Verification items for the finished model (mm, model axes). A direction names the side the tool comes from. Give positions to 0.01 mm unless a question says otherwise; leave off trailing zeros. Loops run counter-clockwise (first coordinate to the right, second up) from the corner with the lowest first, then second, coordinate; pieces in that order, holes last. Notation, with made-up numbers: (46.25, 35.5) - (74.25, 35.5) arc R36 ccw to (74.25, 71.5) - close; hole circle Ø7 at (59, 70.25). An arc over 180 degrees is marked (long way). One line per question, with ' | ' between items. Start each with the question number.
1. Mould release check, pull along X, two halves, no side actions. Record for faces 5 (the face through (10, 175.4, 9.7)), 6 (the face through (-7, 178, -9.5)), 7 (the face through (0, 169, -10)): +X half, -X half, draft (parallel to the pull), parting line (faces both ways), or undercut.
2. Section check B-B, the plane z = 0. Enter the section's corners in (x, y).
3. Section check C-C, the plane y = 100.5. Enter the section's corners in (x, z), then the cut area to 3 significant figures.
4. Section check A-A, the plane y = 174. Enter the section's corners in (x, z).
5. Tool access check on faces 1 (the face through (-7.81, 75.92, -1.73)), 2 (the face through (7, 178, -9.5)), 3 (the face through (-2.4, 173.8, 9)), 4 (the face through (-7.81, 173.76, -1.73)). Record the directions out of +Z, -Z, +X, -X, +Y, -Y that give a thin tool (end or side, any length) a straight path to the whole face; none if there is none.
6. Thickness scan on line 1 along Y through (x, z) = (0, -9.5); line 2 along X through (y, z) = (73, 0); line 3 along X through (y, z) = (155, -1). Record the ranges inside material, lowest first. Write a range as from..to.
7. Depth check by flat-ended pin: pin 1 Ø6 at (x, y) = (2.5, 109) entering from +Z; pin 2 Ø3 at (x, y) = (0, 31.5) entering from -Z; pin 3 Ø9 at (x, z) = (4, 2) entering from +Y; pin 4 Ø4 at (y, z) = (118, -3) entering from -X. Enter the tip coordinate at first touch or a pass-through.
from build123d import *

# Parameters (mm, degrees)
SKETCH1_R           = 8
BOSS_EXTRUDE1_DEPTH = 154
SKETCH2_W           = 20
SKETCH2_H           = 20
BOSS_EXTRUDE2_DEPTH = 40
SKETCH3_W           = 18
SKETCH3_H           = 34
CUT_EXTRUDE1_DEPTH  = 196.28440798
SKETCH6_R           = 8
BOSS_EXTRUDE3_DEPTH = 34
SKETCH7_R           = 3.5
CUT_EXTRUDE4_DEPTH  = 1
CUT_EXTRUDE5_DEPTH  = 1
SKETCH4_R           = 6
CUT_EXTRUDE3_DEPTH  = 195.514780929


with BuildPart() as part:
    # Sketch1 → Boss-Extrude1 (new body)
    with BuildSketch(Plane(origin=(0, 0, 0), x_dir=(1, 0, 0), z_dir=(0, 1, 0))):
        with Locations(Location((0, 0, 0), (0, 0, 270))):
            Circle(SKETCH1_R)
    extrude(amount=BOSS_EXTRUDE1_DEPTH)

    # Sketch2 → Boss-Extrude2 (add)
    with BuildSketch(Plane(origin=(0, 154, 0), x_dir=(1, 0, 0), z_dir=(0, 1, 0))):
        Rectangle(SKETCH2_W, SKETCH2_H)
    extrude(amount=BOSS_EXTRUDE2_DEPTH)

    # Sketch3 → Cut-Extrude1 (cut, through all)
    with BuildSketch(Plane.ZY.offset(10)):
        with Locations((0, 174)):
            Rectangle(SKETCH3_W, SKETCH3_H)
    extrude(amount=-CUT_EXTRUDE1_DEPTH, mode=Mode.SUBTRACT)

    # Sketch6 → Boss-Extrude3 (add)
    with BuildSketch(Plane(origin=(0, 157, 0), x_dir=(1, 0, 0), z_dir=(0, 1, 0))):
        with Locations(Location((0, 0, 0), (0, 0, 270))):
            Circle(SKETCH6_R)
    extrude(amount=BOSS_EXTRUDE3_DEPTH)

    # Sketch7 → Cut-Extrude4 (cut)
    with BuildSketch(Plane(origin=(0, 0, -10), x_dir=(-1, 0, 0), z_dir=(0, 0, -1))):
        with Locations((0, 174)):
            Circle(SKETCH7_R)
        with BuildLine():
            Line((-0.25, 178), (0.25, 178))
            ThreePointArc((0.25, 178), (0.780330086, 178.219669914), (1, 178.75))
            Line((1, 178.75), (1, 185.25))
            ThreePointArc((1, 185.25), (0.780330086, 185.780330086), (0.25, 186))
            Line((0.25, 186), (-0.25, 186))
            ThreePointArc((-0.25, 186), (-0.780330086, 185.780330086), (-1, 185.25))
            Line((-1, 185.25), (-1, 178.75))
            ThreePointArc((-1, 178.75), (-0.780330086, 178.219669914), (-0.25, 178))
        make_face()
        with BuildLine():
            Line((-4.4, 176.05), (-9.6, 179.95))
            ThreePointArc((-9.6, 179.95), (-9.89246212, 180.443933983), (-9.75, 181))
            Line((-9.75, 181), (-9.45, 181.4))
            ThreePointArc((-9.45, 181.4), (-8.956066017, 181.69246212), (-8.4, 181.55))
            Line((-8.4, 181.55), (-3.2, 177.65))
            ThreePointArc((-3.2, 177.65), (-2.90753788, 177.156066017), (-3.05, 176.6))
            Line((-3.05, 176.6), (-3.35, 176.2))
            ThreePointArc((-3.35, 176.2), (-3.843933983, 175.90753788), (-4.4, 176.05))
        make_face()
        with BuildLine():
            Line((3.2, 177.65), (8.4, 181.55))
            ThreePointArc((8.4, 181.55), (8.956066017, 181.69246212), (9.45, 181.4))
            Line((9.45, 181.4), (9.75, 181))
            ThreePointArc((9.75, 181), (9.89246212, 180.443933983), (9.6, 179.95))
            Line((9.6, 179.95), (4.4, 176.05))
            ThreePointArc((4.4, 176.05), (3.843933983, 175.90753788), (3.35, 176.2))
            Line((3.35, 176.2), (3.05, 176.6))
            ThreePointArc((3.05, 176.6), (2.90753788, 177.156066017), (3.2, 177.65))
        make_face()
        with BuildLine():
            Line((3.35, 263.8), (3.05, 263.4))
            ThreePointArc((3.05, 263.4), (2.90753788, 262.843933983), (3.2, 262.35))
            Line((3.2, 262.35), (8.4, 258.45))
            ThreePointArc((8.4, 258.45), (8.956066017, 258.30753788), (9.45, 258.6))
            Line((9.45, 258.6), (9.75, 259))
            ThreePointArc((9.75, 259), (9.89246212, 259.556066017), (9.6, 260.05))
            Line((9.6, 260.05), (4.4, 263.95))
            ThreePointArc((4.4, 263.95), (3.843933983, 264.09246212), (3.35, 263.8))
        make_face()
        with BuildLine():
            Line((-3.05, 263.4), (-3.35, 263.8))
            ThreePointArc((-3.35, 263.8), (-3.843933983, 264.09246212), (-4.4, 263.95))
            Line((-4.4, 263.95), (-9.6, 260.05))
            ThreePointArc((-9.6, 260.05), (-9.89246212, 259.556066017), (-9.75, 259))
            Line((-9.75, 259), (-9.45, 258.6))
            ThreePointArc((-9.45, 258.6), (-8.956066017, 258.30753788), (-8.4, 258.45))
            Line((-8.4, 258.45), (-3.2, 262.35))
            ThreePointArc((-3.2, 262.35), (-2.90753788, 262.843933983), (-3.05, 263.4))
        make_face()
        with BuildLine():
            Line((1, 261.25), (1, 254.75))
            ThreePointArc((1, 254.75), (0.780330086, 254.219669914), (0.25, 254))
            Line((0.25, 254), (-0.25, 254))
            ThreePointArc((-0.25, 254), (-0.780330086, 254.219669914), (-1, 254.75))
            Line((-1, 254.75), (-1, 261.25))
            ThreePointArc((-1, 261.25), (-0.780330086, 261.780330086), (-0.25, 262))
            Line((-0.25, 262), (0.25, 262))
            ThreePointArc((0.25, 262), (0.780330086, 261.780330086), (1, 261.25))
        make_face()
    extrude(amount=-CUT_EXTRUDE4_DEPTH, mode=Mode.SUBTRACT)

    # Sketch8 → Cut-Extrude5 (cut)
    with BuildSketch(Plane.XY.offset(10)):
        with BuildLine():
            Line((-0.5, 158), (0.5, 158))
            ThreePointArc((0.5, 158), (1.560660172, 158.439339828), (2, 159.5))
            Line((2, 159.5), (2, 188.5))
            ThreePointArc((2, 188.5), (1.560660172, 189.560660172), (0.5, 190))
            Line((0.5, 190), (-0.5, 190))
            ThreePointArc((-0.5, 190), (-1.560660172, 189.560660172), (-2, 188.5))
            Line((-2, 188.5), (-2, 159.5))
            ThreePointArc((-2, 159.5), (-1.560660172, 158.439339828), (-0.5, 158))
        make_face()
        with BuildLine():
            Line((-6.932239868, 160), (-5.932239868, 160))
            ThreePointArc((-5.932239868, 160), (-4.871579696, 160.439339828), (-4.432239868, 161.5))
            Line((-4.432239868, 161.5), (-4.432239868, 186.5))
            ThreePointArc((-4.432239868, 186.5), (-4.871579696, 187.560660172), (-5.932239868, 188))
            Line((-5.932239868, 188), (-6.932239868, 188))
            ThreePointArc((-6.932239868, 188), (-7.992900039, 187.560660172), (-8.432239868, 186.5))
            Line((-8.432239868, 186.5), (-8.432239868, 161.5))
            ThreePointArc((-8.432239868, 161.5), (-7.992900039, 160.439339828), (-6.932239868, 160))
        make_face()
        with BuildLine():
            Line((4.432239868, 161.5), (4.432239868, 186.5))
            ThreePointArc((4.432239868, 186.5), (4.871579696, 187.560660172), (5.932239868, 188))
            Line((5.932239868, 188), (6.932239868, 188))
            ThreePointArc((6.932239868, 188), (7.992900039, 187.560660172), (8.432239868, 186.5))
            Line((8.432239868, 186.5), (8.432239868, 161.5))
            ThreePointArc((8.432239868, 161.5), (7.992900039, 160.439339828), (6.932239868, 160))
            Line((6.932239868, 160), (5.932239868, 160))
            ThreePointArc((5.932239868, 160), (4.871579696, 160.439339828), (4.432239868, 161.5))
        make_face()
    extrude(amount=-CUT_EXTRUDE5_DEPTH, mode=Mode.SUBTRACT)

    # Sketch4 → Cut-Extrude3 (cut, through all)
    with BuildSketch(Plane(origin=(0, 194, 0), x_dir=(1, 0, 0), z_dir=(0, 1, 0))):
        with Locations(Location((0, 0, 0), (0, 0, 270))):
            Circle(SKETCH4_R)
    extrude(amount=-CUT_EXTRUDE3_DEPTH, mode=Mode.SUBTRACT)


solid = part.part
Results list:
1) face 5: +X half | face 6: undercut | face 7: draft
2) outline: (-10, 154) - (-8, 154) - (-8, 0) - (-6, 0) - (-6, 194) - (-10, 194) - (-10, 191) - (-8, 191) - (-8, 157) - (-10, 157) - close; (6, 0) - (8, 0) - (8, 154) - (10, 154) - (10, 157) - (8, 157) - (8, 191) - (10, 191) - (10, 194) - (6, 194) - close
3) outline: circle Ø16 at (0, 0); hole circle Ø12 at (0, 0) | area: 88.0 mm²
4) outline: (-10, -10) - (-3.5, -10) - (-3.5, -9) - (-10, -9) - close; (-10, 9) - (-8.43, 9) - (-8.43, 10) - (-10, 10) - close; circle Ø16 at (0, 0); (-4.43, 9) - (-2, 9) - (-2, 10) - (-4.43, 10) - close; (2, 9) - (4.43, 9) - (4.43, 10) - (2, 10) - close; (3.5, -10) - (10, -10) - (10, -9) - (3.5, -9) - close; (8.43, 9) - (10, 9) - (10, 10) - (8.43, 10) - close; hole circle Ø12 at (0, 0)
5) face 1: -Y | face 2: -Z | face 3: +X, -X | face 4: none
6) line 1: 154..170.5, 177.5..178, 186..194 | line 2: -8..-6, 6..8 | line 3: -10..-5.92, 5.92..10
7) pin 1: z = 8 | pin 2: z = -8 | pin 3: y = 194 | pin 4: x = -7.94
